```python
from build123d import *

# Parameters (mm, degrees)
F1_DEPTH = 3.175
F4_DEPTH = 76.2
F5_DEPTH = 43.942


with BuildPart() as f1:
    # F0 (on Front) → F1 (new body)
    with BuildSketch(Plane.XZ):
        Polygon((-34.925, -57.010706), (9.447175, -57.010706), (14.970036, -32.218409), (18.069073, -32.908767), (20.830503, -20.512618), (17.731466, -19.82226), (26.562884, 19.82226), (29.661922, 19.131903), (32.423352, 31.528051), (29.324315, 32.218409), (34.847175, 57.010706), (-34.925, 57.010706), (-34.925, 31.610706), (-38.1, 31.610706), (-38.1, 18.910706), (-34.925, 18.910706), (-34.925, -18.910706), (-38.1, -18.910706), (-38.1, -31.610706), (-34.925, -31.610706), align=None)
    extrude(amount=F1_DEPTH)

    # F3 (on face) → F4 (cut)
    with BuildSketch(Plane(origin=(-34.925, 0, 0), x_dir=(0, -1, 0), z_dir=(-1, 0, 0))):
        Polygon((3.175, 57.010706), (0, 57.010706), (3.175, 55.393441), align=None)
    extrude(amount=-F4_DEPTH, mode=Mode.SUBTRACT)

    # F2 (on face) → F5 (join)
    with BuildSketch(Plane(origin=(-34.925, 0, 0), x_dir=(0, -1, 0), z_dir=(-1, 0, 0))):
        Polygon((-5.658236, -54.128543), (0, -57.010706), (3.175, -58.627972), (3.175, -55.064803), (-4.217154, -51.299425), align=None)
    extrude(amount=-F5_DEPTH)


solid = f1.part
```
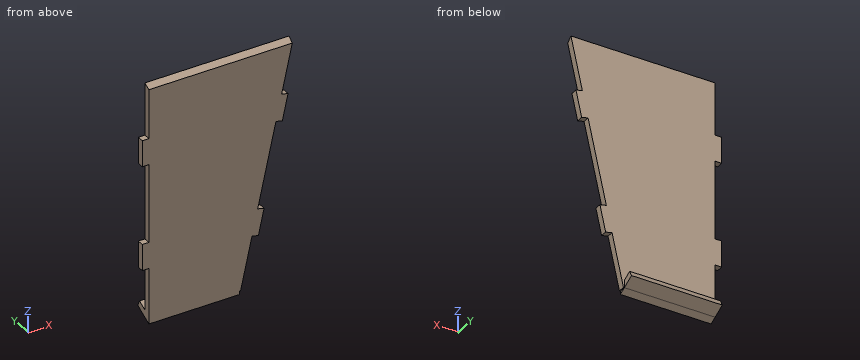
Verification items for the finished model (mm, model axes). Coordinates: 2 decimals unless noted, no trailing zeros. Write each loop counter-clockwise with the first axis right and the second up, starting at its lowest first coordinate (ties: lowest second). Pieces come first, ordered by that corner, then holes. Notation, with made-up numbers: (-19, -22.75) - (-13, -22.75) arc R20 cw to (-13, -5.75) - close; hole circle Ø1 at (27, 32.25). An arc over 180 degrees is marked (long way). One line per question, with ' | ' between items. Start each with the question number.
1. Section check A-A (x = -5.5). Enter the section's corners in (y, z) (3 decimals), plus the area to 3 significant figures.
2. Gauge pin test, flat ends, axial feed: P1, Ø3.5, axis at y = -2, z = -7.5, coming from the -X side (3 decimals); P2, Ø0.8, axis at y = -2, z = -58, coming from the +X side; P3, Ø3.5, axis at x = -37, y = -2, coming from the +Z side. Record the tip position at first contact, or that the pin passes through.
3. Section check D-D (z = -42.5). Enter the section's corners in (x, y) (3 decimals), plus the area to 3 significant figures.
4. Section check C-C (z = -25.5). Enter the section's corners in (x, y) (3 decimals), plus the area to 3 significant figures.
5. Section check B-B (y = -1.75). Enter the section's corners in (x, z) (1 decimal).
6. Material ranges on line 1 along Y through (x, z) = (7.5, 48) (3 decimals); line 2 along Z through (x, y) = (-32.5, 4.5); line 3 along Z through (x, y) = (6, -0.5), recorded low to high.
Computed values:
1) outline: (-3.175, -58.628) - (0, -57.011) - (5.658, -54.129) - (4.217, -51.299) - (0, -53.448) - (0, 57.011) - (-3.175, 55.393) - close | area: 380 mm²
2) P1: x = -34.925 | P2: x = 9.02 | P3: z = 31.61
3) outline: (-34.925, -3.175) - (12.68, -3.175) - (12.68, 0) - (-34.925, 0) - close | area: 151 mm²
4) outline: (-38.1, -3.175) - (19.719, -3.175) - (19.719, 0) - (-38.1, 0) - close | area: 184 mm²
5) outline: (-38.1, -31.6) - (-34.9, -31.6) - (-34.9, -57.9) - (9, -57.9) - (9, -57) - (9.4, -57) - (15, -32.2) - (18.1, -32.9) - (20.8, -20.5) - (17.7, -19.8) - (26.6, 19.8) - (29.7, 19.1) - (32.4, 31.5) - (29.3, 32.2) - (34.6, 56.1) - (-34.9, 56.1) - (-34.9, 31.6) - (-38.1, 31.6) - (-38.1, 18.9) - (-34.9, 18.9) - (-34.9, -18.9) - (-38.1, -18.9) - close
6) line 1: -3.175 to 0 | line 2: -54.72 to -51.85 | line 3: -57.27 to 56.76
